Design review of the part built by this model. Coordinates are the model's own, in mm. Face numbers are marked on the shaded views. Round coordinates to 2 decimals unless told otherwise and drop trailing zeros. Loops run counter-clockwise (first coordinate to the right, second up) from the corner with the lowest first, then second, coordinate; pieces in that order, holes last. Notation, with made-up numbers: (-35, 65) -> (18, 65) arc R28 cw to (18, 103) -> close; hole circle Ø10 at (59, 36). An arc over 180 degrees is marked (long way). Write each question's results on one line, items separated by ' | '. Start each with the question number.
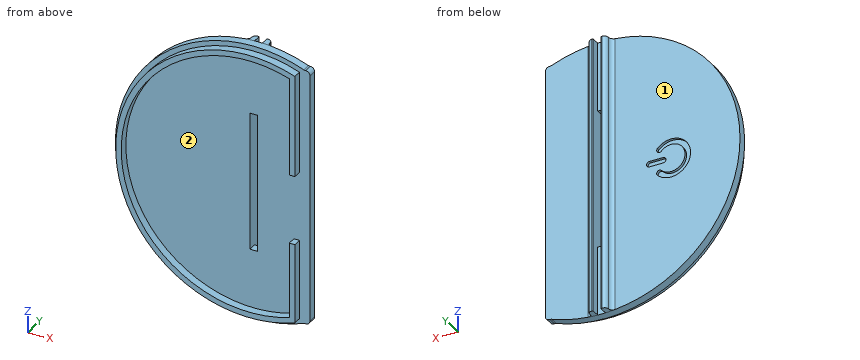
from build123d import *
from build123d.topology import SkipClean

# Parameters (mm, degrees)
BOSS_EXTRUDE1_DEPTH     = 3
CUT_EXTRUDE1_DEPTH      = 71.774289117
CUT_EXTRUDE1_DEPTH_BACK = 71.774289117
SKETCH2_W               = 2.8
SKETCH2_H               = 50
BOSS_EXTRUDE2_DEPTH     = 3
SKETCH4_W               = 2
SKETCH4_H               = 25
CUT_EXTRUDE2_DEPTH      = 3
BOSS_EXTRUDE3_DEPTH     = 3
SKETCH7_W               = 93.053616802
SKETCH7_H               = 3
BOSS_EXTRUDE4_DEPTH     = 2
CUT_EXTRUDE3_DEPTH      = 1
FILLET1_R               = 1.5


with BuildPart() as part:
    # Sketch1 → Boss-Extrude1 (new body)
    with BuildSketch(Plane(origin=(0, 0, 0), x_dir=(1, 0, 0), z_dir=(0, 1, 0))):
        with BuildLine():
            Line((18.31, 46.526808401), (18.31, -46.526808401))
            ThreePointArc((18.31, -46.526808401), (-50, 0), (18.31, 46.526808401))
        make_face()
    extrude(amount=BOSS_EXTRUDE1_DEPTH)

    # Sketch2 → Cut-Extrude1 (cut, two sides: drawn at the far end of the back side and taken through both)
    with BuildSketch(Plane(origin=(0, 3, 0), x_dir=(1, 0, 0), z_dir=(0, 1, 0)).offset(-CUT_EXTRUDE1_DEPTH_BACK)):
        Rectangle(SKETCH2_W, SKETCH2_H)
    extrude(amount=CUT_EXTRUDE1_DEPTH + CUT_EXTRUDE1_DEPTH_BACK, mode=Mode.SUBTRACT)

    # Sketch3 → Boss-Extrude2 (add)
    with BuildSketch(Plane.XZ):
        with BuildLine():
            Line((16.51, -45.284212481), (16.51, 45.284212481))
            ThreePointArc((16.51, 45.284212481), (-48.2, 0), (16.51, -45.284212481))
        make_face()
        with BuildLine():
            Line((14.51, -43.862283342), (14.51, 43.862283342))
            ThreePointArc((14.51, 43.862283342), (-46.2, 0), (14.51, -43.862283342))
        make_face(mode=Mode.SUBTRACT)
    extrude(amount=BOSS_EXTRUDE2_DEPTH)

    # Sketch4 → Cut-Extrude2 (cut)
    with BuildSketch(Plane.XZ.offset(3)):
        with Locations((15.51, -4.026808401)):
            Rectangle(SKETCH4_W, SKETCH4_H)
    extrude(amount=-CUT_EXTRUDE2_DEPTH, mode=Mode.SUBTRACT)

    # Sketch6 → Boss-Extrude3 (add)
    with SkipClean():  # the faces are left unmerged after this step: merging them gives an invalid solid
        with BuildSketch(Plane(origin=(0, 3, 0), x_dir=(1, 0, 0), z_dir=(0, 1, 0))):
            with BuildLine():
                Line((-1.4, 25), (-1.4, 49.980396157))
                ThreePointArc((-1.4, 49.980396157), (-2.400481254, 49.942343655), (-3.4, 49.884266057))
                Line((-3.4, 49.884266057), (-3.4, -49.884266057))
                ThreePointArc((-3.4, -49.884266057), (-2.400481254, -49.942343655), (-1.4, -49.980396157))
                Line((-1.4, -49.980396157), (-1.4, -25))
                Line((-1.4, -25), (-1.4, 25))
            make_face()
            with BuildLine():
                ThreePointArc((3.4, 49.884266057), (2.400481254, 49.942343655), (1.4, 49.980396157))
                Line((1.4, 49.980396157), (1.4, 25))
                Line((1.4, 25), (1.4, -25))
                Line((1.4, -25), (1.4, -49.980396157))
                ThreePointArc((1.4, -49.980396157), (2.400481254, -49.942343655), (3.4, -49.884266057))
                Line((3.4, -49.884266057), (3.4, 49.884266057))
            make_face()
        extrude(amount=BOSS_EXTRUDE3_DEPTH)

    # Sketch7 → Boss-Extrude4 (add)
    with SkipClean():  # the faces are left unmerged after this step: merging them gives an invalid solid
        with BuildSketch(Plane(origin=(18.31, 0, 0), x_dir=(0, 0, -1), z_dir=(1, 0, 0))):
            with Locations((0, 1.5)):
                Rectangle(SKETCH7_W, SKETCH7_H)
        extrude(amount=BOSS_EXTRUDE4_DEPTH)

    # Sketch8 → Cut-Extrude3 (cut)
    with SkipClean():  # the faces are left unmerged after this step: merging them gives an invalid solid
        with BuildSketch(Plane(origin=(0, 3, 0), x_dir=(1, 0, 0), z_dir=(0, 1, 0))):
            with BuildLine():
                Line((-17.253164172, 1), (-22.253164172, 1))
                ThreePointArc((-22.253164172, 1), (-23.253164172, 0), (-22.253164172, -1))
                Line((-22.253164172, -1), (-17.253164172, -1))
                ThreePointArc((-17.253164172, -1), (-16.253164172, 0), (-17.253164172, 1))
            make_face()
            with BuildLine():
                ThreePointArc((-20.190928157, 4.949747468), (-32.140675626, 0), (-20.190928157, -4.949747468))
                ThreePointArc((-20.190928157, -4.949747468), (-20.190928157, -3.535533906), (-21.60514172, -3.535533906))
                ThreePointArc((-21.60514172, -3.535533906), (-30.140675626, 0), (-21.60514172, 3.535533906))
                ThreePointArc((-21.60514172, 3.535533906), (-20.190928157, 3.535533906), (-20.190928157, 4.949747468))
            make_face()
        extrude(amount=-CUT_EXTRUDE3_DEPTH, mode=Mode.SUBTRACT)

    # Fillet1
    # the kernel refuses this fillet: 1.5 mm, written as the material it adds along each edge
    with BuildSketch(Plane(origin=(18.31, 0, -46.526808401), x_dir=(-0.9315513824511361, 0, -0.3636097108898181), z_dir=(0, 1, 0))) as fillet1_piece_1:
        with BuildLine():
            CenterArc((0.282386116, -1.499994195), FILLET1_R, 90.159404468, 21.162642488)
            Line((-0.26302845, -0.102667121), (0, 0))
            ThreePointArc((0, 0), (0.139106461, -0.000193506), (0.278212923, 0))
        make_face()
    extrude(amount=3)
    with BuildSketch(Plane(origin=(18.31, 0, 46.526808401), x_dir=(-0.9315513824511399, 0, 0.3636097108898083), z_dir=(0, 1, 0))) as fillet1_piece_2:
        with BuildLine():
            CenterArc((0.282386116, 1.499994195), FILLET1_R, 248.677953043, 21.162642488)
            Line((-0.26302845, 0.102667121), (0, 0))
            ThreePointArc((0, 0), (0.139106461, 0.000193506), (0.278212923, 0))
        make_face()
    extrude(amount=3)
    with BuildSketch(Plane(origin=(-3.4, 3, -53.634266057), x_dir=(-1, 0, 0), z_dir=(0, 0, 1))) as fillet1_piece_3_section:
        with BuildLine():
            CenterArc((FILLET1_R, -FILLET1_R), FILLET1_R, 90, 90)
            Line((0, -FILLET1_R), (0, 0))
            Line((0, 0), (FILLET1_R, 0))
        make_face()
    fillet1_piece_3 = extrude(amount=107.268532113, mode=Mode.PRIVATE)
    fillet1_piece_3 = fillet1_piece_3 & Plane(origin=(0, 3.339687762, 0), x_dir=(0.36619999999999997, 0, 0.9305361680235755), z_dir=(0, -1, 0)) * Cylinder(50, 221, mode=Mode.PRIVATE)
    add(fillet1_piece_3)
    with BuildSketch(Plane(origin=(3.4, 3, 53.634266057), x_dir=(1, 0, 0), z_dir=(0, 0, -1))) as fillet1_piece_4_section:
        with BuildLine():
            CenterArc((FILLET1_R, -FILLET1_R), FILLET1_R, 90, 90)
            Line((0, -FILLET1_R), (0, 0))
            Line((0, 0), (FILLET1_R, 0))
        make_face()
    fillet1_piece_4 = extrude(amount=107.268532113, mode=Mode.PRIVATE)
    fillet1_piece_4 = fillet1_piece_4 & Plane(origin=(0, 3.339687762, 0), x_dir=(0.36619999999999997, 0, 0.9305361680235755), z_dir=(0, -1, 0)) * Cylinder(50, 221, mode=Mode.PRIVATE)
    add(fillet1_piece_4)
    # the kernel refuses this fillet: 1.5 mm, written as the material it takes off along each edge
    with BuildSketch(Plane(origin=(-3.4, 6, -53.634266057), x_dir=(0, -1, 0), z_dir=(0, 0, 1)), Plane(origin=(3.4, 6, 53.634266057), x_dir=(0, -1, 0), z_dir=(0, 0, -1))) as fillet1_2_piece_1:
        with BuildLine():
            CenterArc((FILLET1_R, FILLET1_R), FILLET1_R, 180, 90)
            Line((0, FILLET1_R), (0, 0))
            Line((0, 0), (FILLET1_R, 0))
        make_face()
    extrude(amount=107.268532113, mode=Mode.SUBTRACT)
    with BuildSketch(Plane(origin=(20.31, -3.75, 46.526808401), x_dir=(-1, 0, 0), z_dir=(0, 1, 0)), Plane(origin=(20.31, 6.75, -46.526808401), x_dir=(-1, 0, 0), z_dir=(0, -1, 0))) as fillet1_2_piece_2:
        with BuildLine():
            CenterArc((FILLET1_R, -FILLET1_R), FILLET1_R, 90, 90)
            Line((0, -FILLET1_R), (0, 0))
            Line((0, 0), (FILLET1_R, 0))
        make_face()
    extrude(amount=10.5, mode=Mode.SUBTRACT)


solid = part.part
1) The part is to be moulded in two halves that separate along X. For the marked faces 1 and 2, say which applies: +X half, -X half, draft (parallel to the pull), parting line (faces both ways), or undercut.
2) Take a section at D-D (z = 10). Write out the cut boundary in (x, y).
3) Insertion check: pin 1 (5 mm diameter, centred on y = 2, z = -27.5, fed in from -X); pin 2 (2.5 mm diameter, centred on y = -1, z = 18, fed in from -X); pin 3 (0.9 mm diameter, centred on y = -1, z = -36.5, fed in from -X). Each pin has a flat end and moves straight along its axis. Give the tip position at first contact, or say it passes through.
4) Take a section at A-A (x = 0). Write out the cut boundary in (y, z), plus the area to 3 significant figures.
5) Take a section at B-B (z = 0). Write out the cut boundary in (x, y).
6) To check wall thickness, follow line 1 (Z direction, x = 0, y = -1.45); line 2 (X direction, y = -1.9, z = 0); line 3 (Y direction, x = -30, z = -34.5). State the ranges of each line that lie inside material, in increasing order. Write a range as from..to.
7) Take a section at C-C (x = -38). Write out the cut boundary in (y, z).
Geometry check:
1) face 1: draft | face 2: undercut
2) outline: (-48.99, 0) -> (-47.15, 0) -> (-47.15, -3) -> (-45.1, -3) -> (-45.1, 0) -> (-1.4, 0) -> (-1.4, 6) -> (-1.9, 6) arc R1.5 ccw to (-3.4, 4.5) arc R1.5 cw to (-4.9, 3) -> (-48.99, 3) -> close; (1.4, 0) -> (14.51, 0) -> (14.51, -3) -> (16.51, -3) -> (16.51, 0) -> (20.31, 0) -> (20.31, 3) -> (4.9, 3) arc R1.5 cw to (3.4, 4.5) arc R1.5 ccw to (1.9, 6) -> (1.4, 6) -> close
3) pin 1: stops at x = -43.3 | pin 2: stops at x = -46.93 | pin 3: stops at x = -31.99
4) outline: (-3, -48.2) -> (0, -48.2) -> (0, -50) -> (3, -50) -> (3, -25) -> (0, -25) -> (0, -46.2) -> (-3, -46.2) -> close; (-3, 46.2) -> (0, 46.2) -> (0, 25) -> (3, 25) -> (3, 50) -> (0, 50) -> (0, 48.2) -> (-3, 48.2) -> close | area: 162 mm^2
5) outline: (-50, 0) -> (-48.2, 0) -> (-48.2, -3) -> (-46.2, -3) -> (-46.2, 0) -> (-1.4, 0) -> (-1.4, 6) -> (-1.9, 6) arc R1.5 ccw to (-3.4, 4.5) arc R1.5 cw to (-4.9, 3) -> (-16.25, 3) -> (-16.25, 2) -> (-23.25, 2) -> (-23.25, 3) -> (-30.14, 3) -> (-30.14, 2) -> (-32.14, 2) -> (-32.14, 3) -> (-50, 3) -> close; (1.4, 0) -> (20.31, 0) -> (20.31, 3) -> (4.9, 3) arc R1.5 cw to (3.4, 4.5) arc R1.5 ccw to (1.9, 6) -> (1.4, 6) -> close
6) line 1: z = -48.2..-46.2, 46.2..48.2 | line 2: x = -48.2..-46.2 | line 3: y = 0..3
7) outline: (-3, -29.65) -> (0, -29.65) -> (0, -32.5) -> (3, -32.5) -> (3, 32.5) -> (0, 32.5) -> (0, 29.65) -> (-3, 29.65) -> (-3, 26.28) -> (0, 26.28) -> (0, -26.28) -> (-3, -26.28) -> close
